Build history of the part. All positions in model axes, mm. Face numbers are marked on the shaded views. A direction names the side the tool comes from. Round coordinates to 2 decimals unless told otherwise and drop trailing zeros. Write each loop counter-clockwise with the first axis right and the second up, starting at its lowest first coordinate (ties: lowest second). Pieces come first, ordered by that corner, then holes.
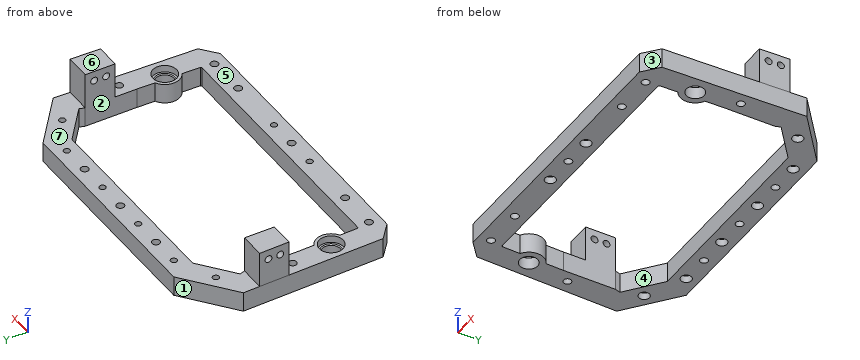
from build123d import *

# Parameters (mm, degrees)
SKETCH1_R               = 6
SKETCH1_R_2             = 1.6
BOSS_EXTRUDE1_DEPTH     = 10
BOSS_EXTRUDE2_DEPTH     = 18
SKETCH7_R               = 1.75
CUT_EXTRUDE4_DEPTH      = 148
CUT_EXTRUDE4_DEPTH_BACK = 14
SKETCH8_R               = 2.65
CUT_EXTRUDE5_DEPTH      = 3.5
BOSS_EXTRUDE3_START     = -10
SKETCH10_R              = 6.870136932
SKETCH10_R_2            = 4.5
SKETCH10_R_3            = 6.9172188
BOSS_EXTRUDE3_DEPTH     = 6.5
SKETCH11_R              = 1.95
CUT_EXTRUDE6_DEPTH      = 29
CHAMFER1_SIZE           = 0.5


with BuildPart() as part:
    # Sketch1 → Boss-Extrude1 (new body)
    with BuildSketch(Plane.XY):
        Polygon((-55.131687722, 48.97503592), (54.868312278, 48.97503592), (79.868312278, 28.97503592), (77.800969503, -42.368674328), (69.868312278, -49.02496408), (-70.131687722, -49.02496408), (-78.064344947, -42.368674328), (-80.131687722, 28.97503592), align=None)
        with Locations((-70.131687722, -21.02496408)):
            Circle(SKETCH1_R, mode=Mode.SUBTRACT)
        with Locations((69.868312278, -21.02496408)):
            Circle(SKETCH1_R, mode=Mode.SUBTRACT)
        with Locations((-45.131687722, 42.97503592)):
            Circle(SKETCH1_R_2, mode=Mode.SUBTRACT)
        with Locations((-15.131687722, 42.97503592)):
            Circle(SKETCH1_R_2, mode=Mode.SUBTRACT)
        with Locations((14.868312278, 42.97503592)):
            Circle(SKETCH1_R_2, mode=Mode.SUBTRACT)
        with Locations((44.868312278, 42.97503592)):
            Circle(SKETCH1_R_2, mode=Mode.SUBTRACT)
        with Locations((-64.740033508, 33.604610207)):
            Circle(SKETCH1_R_2, mode=Mode.SUBTRACT)
        with Locations((64.476658063, 33.604610207)):
            Circle(SKETCH1_R_2, mode=Mode.SUBTRACT)
        with Locations((-15.131687722, -43.02496408)):
            Circle(SKETCH1_R_2, mode=Mode.SUBTRACT)
        with Locations((14.868312278, -43.02496408)):
            Circle(SKETCH1_R_2, mode=Mode.SUBTRACT)
        with BuildLine():
            Line((-67.963425231, 23.342147743), (-50.92231501, 36.97503592))
            Line((-50.92231501, 36.97503592), (50.658939565, 36.97503592))
            Line((50.658939565, 36.97503592), (67.700049787, 23.342147743))
            Line((67.700049787, 23.342147743), (66.868312278, 20.639002542))
            Line((66.868312278, 20.639002542), (66.868312278, -5.360997458))
            Line((66.868312278, -5.360997458), (66.610164686, -14.269634756))
            ThreePointArc((66.610164686, -14.269634756), (62.371459095, -20.807726075), (66.224458755, -27.580292561))
            Line((66.224458755, -27.580292561), (65.961995417, -36.637865644))
            Line((65.961995417, -36.637865644), (65.500669466, -37.02496408))
            Line((65.500669466, -37.02496408), (-65.764044911, -37.02496408))
            Line((-65.764044911, -37.02496408), (-66.225370862, -36.637865644))
            Line((-66.225370862, -36.637865644), (-66.487834199, -27.580292561))
            ThreePointArc((-66.487834199, -27.580292561), (-62.634834539, -20.807726075), (-66.873540131, -14.269634756))
            Line((-66.873540131, -14.269634756), (-67.131687722, -5.360997458))
            Line((-67.131687722, -5.360997458), (-67.131687722, 20.639002542))
            Line((-67.131687722, 20.639002542), (-67.963425231, 23.342147743))
        make_face(mode=Mode.SUBTRACT)
    extrude(amount=BOSS_EXTRUDE1_DEPTH)

    # Sketch5 → Boss-Extrude2 (add)
    with BuildSketch(Plane.XY.offset(10)):
        Polygon((66.868312278, 20.639002542), (79.192098778, 20.639002542), (79.626757159, 20.639002542), (79.192098778, 5.639002542), (66.868312278, 5.639002542), align=None)
        Polygon((-79.890132604, 20.639002542), (-79.455474222, 5.639002542), (-67.131687722, 5.639002542), (-67.131687722, 20.639002542), (-79.455474222, 20.639002542), align=None)
    extrude(amount=BOSS_EXTRUDE2_DEPTH)

    # Sketch7 → Cut-Extrude4 (cut, two sides)
    with BuildSketch(Plane(origin=(-67.131687722, 0, 0), x_dir=(0, 0, -1), z_dir=(1, 0, 0))) as cut_extrude4_sk:
        with Locations((-23, 16.139002542)):
            Circle(SKETCH7_R)
        with Locations((-23, 10.139002542)):
            Circle(SKETCH7_R)
    extrude(amount=CUT_EXTRUDE4_DEPTH, mode=Mode.SUBTRACT)
    extrude(cut_extrude4_sk.sketch, amount=-CUT_EXTRUDE4_DEPTH_BACK, mode=Mode.SUBTRACT)

    # Sketch8 → Cut-Extrude5 (cut)
    with BuildSketch(Plane(origin=(0, 0, 0), x_dir=(-1, 0, 0), z_dir=(0, 0, -1))):
        with Locations((-14.868312278, 42.97503592)):
            Circle(SKETCH8_R)
        with Locations((15.131687722, 42.97503592)):
            Circle(SKETCH8_R)
        with Locations((45.131687722, 42.97503592)):
            Circle(SKETCH8_R)
        with Locations((64.740033508, 33.604610207)):
            Circle(SKETCH8_R)
        with Locations((-64.476658063, 33.604610207)):
            Circle(SKETCH8_R)
        with Locations((-44.868312278, 42.97503592)):
            Circle(SKETCH8_R)
        with Locations((-14.868312278, -43.02496408)):
            Circle(SKETCH8_R)
        with Locations((15.131687722, -43.02496408)):
            Circle(SKETCH8_R)
    extrude(amount=-CUT_EXTRUDE5_DEPTH, mode=Mode.SUBTRACT)

    # Sketch10 → Boss-Extrude3 (add)
    with BuildSketch(Plane.XY.offset(10).offset(BOSS_EXTRUDE3_START)):
        with Locations((-70.131687722, -21.02496408)):
            Circle(SKETCH10_R)
        with Locations((-70.131687722, -21.02496408)):
            Circle(SKETCH10_R_2, mode=Mode.SUBTRACT)
        with Locations((69.868312278, -21.02496408)):
            Circle(SKETCH10_R_3)
        with Locations((69.868312278, -21.02496408)):
            Circle(SKETCH10_R_2, mode=Mode.SUBTRACT)
    extrude(amount=BOSS_EXTRUDE3_DEPTH)

    # Sketch11 → Cut-Extrude6 (cut, through all)
    with BuildSketch(Plane(origin=(0, 0, 0), x_dir=(-1, 0, 0), z_dir=(0, 0, -1))):
        with Locations((-29.868312278, 42.97503592)):
            Circle(SKETCH11_R)
        with Locations((0.131687722, 42.97503592)):
            Circle(SKETCH11_R)
        with Locations((30.131687722, 42.97503592)):
            Circle(SKETCH11_R)
        with Locations((0, -43.02496408)):
            Circle(SKETCH11_R)
        with Locations((-45, -43.02496408)):
            Circle(SKETCH11_R)
        with Locations((45, -43.02496408)):
            Circle(SKETCH11_R)
        with Locations((-65, -43.02496408)):
            Circle(SKETCH11_R)
        with Locations((65, -43.02496408)):
            Circle(SKETCH11_R)
        with Locations((-73, 0)):
            Circle(SKETCH11_R)
        with Locations((73, 0)):
            Circle(SKETCH11_R)
    extrude(amount=-CUT_EXTRUDE6_DEPTH, mode=Mode.SUBTRACT)

    # Chamfer1
    chamfer1_edges = [part.edges().sort_by_distance(p)[0] for p in [
        (65.368312278, -21.02496408, 6.5),
        (-74.631687722, -21.02496408, 6.5),
    ]]
    chamfer(chamfer1_edges, length=CHAMFER1_SIZE)


solid = part.part
1) Slice it at C-C (x = -73). Count the separate pieces of the cut face and the enclosed holes in it, plus the area to 3 significant figures.
Results:
separate pieces: 3
enclosed holes: 2
area: 942 mm2
2) Wall check: L1, parallel to Y at x = 45, z = 3.25; L2, parallel to Y at x = 4.5, z = 7.5; L3, parallel to Y at x = -65, z = 4.25. Give the ranges that are in metal, low to high.
Results:
L1: y = -49.02 to -44.97, -41.07 to -37.02, 36.98 to 40.33, 45.62 to 48.98
L2: y = -49.02 to -37.02, 36.98 to 48.98
L3: y = -49.02 to -44.97, -41.07 to -37.02, -26.49 to -15.56, 25.71 to 32.03, 35.18 to 41.08
3) Slice it at A-A (z = 17.5). Write the cut outline in (x, y), plus the area to 3 significant figures.
Results:
outline: (-79.89, 20.64) - (-79.46, 5.64) - (-67.13, 5.64) - (-67.13, 20.64) - close; (66.87, 5.64) - (79.19, 5.64) - (79.63, 20.64) - (66.87, 20.64) - close
area: 376 mm2
4) Slice it at B-B (x = -7). Write the cut outline in (y, z), plus the area to 3 significant figures.
Results:
outline: (-49.02, 0) - (-37.02, 0) - (-37.02, 10) - (-49.02, 10) - close; (36.98, 0) - (48.98, 0) - (48.98, 10) - (36.98, 10) - close
area: 240 mm2
5) Mould opens along Y. For the marked faces 1, 2 and 3 say: released by +Y, released by -Y, zero draft, split by the parting line, or undercut.
Results:
face 1: released by +Y
face 2: undercut
face 3: released by -Y
6) Pin check, flat tips, straight feed: pin 1 Ø8 at (x, y) = (63, -15) entering from +Z; pin 2 Ø5.5 at (y, z) = (10.14, 23) entering from -X; pin 3 Ø2.5 at (x, y) = (15, -42) entering from -Z. Stop position of each tip, or through.
Results:
pin 1: stops at z = 10
pin 2: stops at x = -79.67
pin 3: stops at z = 3.5
7) Which spindle directions (+Z, -Z, +X, -X, +Y, -Y) get a long thin tool onto all of the face, cutting with end or side? Do the marked faces 4, 5, 6 and 7. Say none if no direction does.
Results:
face 4: +Z, -Z
face 5: +Z, +X, -X, -Y
face 6: +Z, +X, -X, +Y, -Y
face 7: +Z, +X, -X, +Y
